Read the model definition and answer for the solid it produces. Units are mm, in the model's axes. A direction names the side the tool comes from. Coordinates: 2 decimals unless noted, no trailing zeros. Write each loop counter-clockwise with the first axis right and the second up, starting at its lowest first coordinate (ties: lowest second). Pieces come first, ordered by that corner, then holes. Notation, with made-up numbers: (27, -14.75) -> (85, -14.75) arc R18 ccw to (85, -6.75) -> close; hole circle Ø11 at (74.25, -31). An arc over 180 degrees is marked (long way). Write item = value, one per line. Start each with the question number.
1) Section A-A (z = 0) is taken. Determine the outline of the cut face in (x, y).
2) Find the intervals of material crossed by line 1 along Z through (x, y) = (-20, 13.5); line 2 along Y through (x, z) = (-20, 2.5); line 3 along Z through (x, y) = (-22.7, -14.25), in increasing order. Write a range as from..to.
3) A tool of negligible diameter and unlimited length cuts with its end or side. For faces 4 (the face through (-13, -7, 23)), 5 (the face through (-18.5, 13.5, 27.5)), 6 (the face through (-15.788, -12.981, -22.242)), from which of +Z, -Z, +X, -X, +Y, -Y can it reach the whole face along a straight path? Write none if from no direction.
4) Section B-B (y = 0) is taken. Determine the outline of the cut face in (x, z), plus the area to 4 significant figures.
5) For a pull along Z with two mould halves and no side action, classify faces 1 (the face through (-21.29, 15.28, -29.32)), 2 (the face through (5.759, 2.994, -22.804)), 3 (the face through (24, -10, -5)) as released by +Z, released by -Z, zero draft, split by the parting line, or undercut.
6) Flat-ended cylindrical pins translate along their axes: pin 1 Ø7 at (y, z) = (28.5, 0) entering from -X; pin 2 Ø8 at (x, z) = (-12.5, -6.5) entering from +Y; pin 3 Ø1.5 at (x, y) = (18, 4.5) entering from +Z; pin 4 Ø10.5 at (y, z) = (-15, -23.5) entering from -X. Find the tip coordinate at first contact, or state that the pin passes through.
7) Section C-C (z = -26) is taken. Determine the outline of the cut face in (x, y), plus the area to 3 significant figures.
8) Section D-D (y = 13) is taken. Determine the outline of the cut face in (x, z).
from build123d import *

# Parameters (mm, degrees)
CUT_EXTRUDE1_REACH = 70.443
SKETCH2_R          = 2.75
SKETCH3_R          = 4.75
CUT_EXTRUDE2_DEPTH = 5.5
CIRPATTERN1_COUNT  = 6


with BuildPart() as part:
    # Sketch1 → Revolve1 (revolve)
    with BuildSketch(Plane.XY, mode=Mode.PRIVATE) as revolve1_sk:
        Polygon((-24, 34.5), (-13, 34.5), (-13, 23), (24, 23), (24, 11), (-24, 11), align=None)
    revolve(revolve1_sk.sketch.rotate(Axis((-82.106015927, 0, 0), (1, 0, 0)), 180), axis=Axis((-82.106015927, 0, 0), (1, 0, 0)))

    # Sketch2 → Cut-Extrude1 (cut, up to next)
    with BuildSketch(Plane.ZY.offset(24), mode=Mode.PRIVATE) as cut_extrude1_sk1:
        with Locations(Location((0, -28.5, 0), (0, 0, 270))):
            Circle(SKETCH2_R)
    cut_extrude1_tool1 = extrude(cut_extrude1_sk1.sketch, amount=-CUT_EXTRUDE1_REACH, mode=Mode.PRIVATE) & part.part
    cut_extrude1 = cut_extrude1_tool1.solids().sort_by_distance((-24, -28.5, 0))[0]
    add(cut_extrude1, mode=Mode.SUBTRACT)

    # Sketch3 → Cut-Extrude2 (cut)
    with BuildSketch(Plane.ZY.offset(24)):
        with Locations(Location((0, -28.5, 0), (0, 0, 270))):
            Circle(SKETCH3_R)
    cut_extrude2 = extrude(amount=-CUT_EXTRUDE2_DEPTH, mode=Mode.SUBTRACT)

    # CirPattern1: Cut-Extrude1, Cut-Extrude2 ×6 about axis
    cirpattern1_axis = Axis((0, 0, 0), (1, 0, 0))
    add([cut_extrude1.rotate(cirpattern1_axis, i * 360 / CIRPATTERN1_COUNT) for i in range(1, CIRPATTERN1_COUNT)], mode=Mode.SUBTRACT)
    add([cut_extrude2.rotate(cirpattern1_axis, i * 360 / CIRPATTERN1_COUNT) for i in range(1, CIRPATTERN1_COUNT)], mode=Mode.SUBTRACT)


solid = part.part
Answer key:
q1.outline = (-24, -34.5) -> (-13, -34.5) -> (-13, -31.25) -> (-18.5, -31.25) -> (-18.5, -33.25) -> (-24, -33.25) -> close; (-24, -23.75) -> (-18.5, -23.75) -> (-18.5, -25.75) -> (-13, -25.75) -> (-13, -23) -> (24, -23) -> (24, -11) -> (-24, -11) -> close; (-24, 11) -> (24, 11) -> (24, 23) -> (-13, 23) -> (-13, 25.75) -> (-18.5, 25.75) -> (-18.5, 23.75) -> (-24, 23.75) -> close; (-24, 33.25) -> (-18.5, 33.25) -> (-18.5, 31.25) -> (-13, 31.25) -> (-13, 34.5) -> (-24, 34.5) -> close
q2.line_1 = -31.75..-29.37, -19.99..19.99, 29.37..31.75
q2.line_2 = -34.41..-32.54, -24.46..-10.71, 10.71..24.46, 32.54..34.41
q2.line_3 = -31.42..-29.43, -19.93..19.93, 29.43..31.42
q3.face_4 = +X
q3.face_5 = -X
q3.face_6 = +X, -X
q4.outline = (-24, -34.5) -> (-13, -34.5) -> (-13, -23) -> (24, -23) -> (24, -11) -> (-24, -11) -> close; (-24, 11) -> (24, 11) -> (24, 23) -> (-13, 23) -> (-13, 34.5) -> (-24, 34.5) -> close
q4.area = 1,405 mm^2
q5.face_1 = undercut
q5.face_2 = split by the parting line
q5.face_3 = zero draft
q6.pin_1 = -18.5
q6.pin_2 = 34.41
q6.pin_3 = 22.69
q6.pin_4 = -24
q7.outline = (-24, -22.68) -> (-13, -22.68) -> (-13, -16.66) -> (-18.5, -16.66) -> (-18.5, -18.81) -> (-24, -18.81) -> close; (-24, -9.69) -> (-18.5, -9.69) -> (-18.5, -11.84) -> (-13, -11.84) -> (-13, 11.84) -> (-18.5, 11.84) -> (-18.5, 9.69) -> (-24, 9.69) -> close; (-24, 18.81) -> (-18.5, 18.81) -> (-18.5, 16.66) -> (-13, 16.66) -> (-13, 22.68) -> (-24, 22.68) -> close
q7.area = 345 mm^2
q8.outline = (-24, -31.96) -> (-13, -31.96) -> (-13, -27.13) -> (-18.5, -27.13) -> (-18.5, -29.26) -> (-24, -29.26) -> close; (-24, -20.1) -> (-18.5, -20.1) -> (-18.5, -22.23) -> (-13, -22.23) -> (-13, -18.97) -> (24, -18.97) -> (24, 18.97) -> (-13, 18.97) -> (-13, 22.23) -> (-18.5, 22.23) -> (-18.5, 20.1) -> (-24, 20.1) -> close; (-24, 29.26) -> (-18.5, 29.26) -> (-18.5, 27.13) -> (-13, 27.13) -> (-13, 31.96) -> (-24, 31.96) -> close
